Can you work these out from the model? Positions are in its coordinate system, mm. Face numbers are marked on the shaded views. A direction names the side the tool comes from. Coordinates: 2 decimals unless noted, no trailing zeros. Order: outer loops, then holes, each group sorted by start corner. A loop starts at its lowest first (then second) coordinate and runs counter-clockwise, first axis right, second up. Notation, with made-up numbers: M 48.5,61 L 59.5,61 A27 cw 59.5,77 Z; hole C 32,1 d5. An arc over 180 degrees is marked long. Answer as CSV lines item,"result". Start each with the question number.
1. If we section it at A-A (z = 4): List the corners of the cut face in (x, y) for me, plus the area to 3 significant figures.
2. On a 3-axis mill with a long thin cutter (end or side, diameter ignored), from which of +Z, -Z, +X, -X, +Y, -Y can I reach the whole of each face in a straight line? I mean the marked faces 1 and 2. Say none if no direction works.
3. If we section it at C-C (y = 23.5): List the corners of the cut face in (x, z) for me, plus the area to 3 significant figures.
4. If we section it at B-B (x = 30): List the corners of the cut face in (y, z) for me.
5. I need wall thicknesses on line 1 along Y through (x, z) = (38.5, 9.25); line 2 along X through (y, z) = (12.5, 11). Which ranges of each line are inside material? Lowest first, please. Write a range as from..to.
6. Will these pins go through, and if not, where does the flat tip stop? pin 1 (5 mm diameter, centred on x = 43, z = 10.5, fed in from -Y); pin 2 (6 mm diameter, centred on y = 5.5, z = 8, fed in from -X).
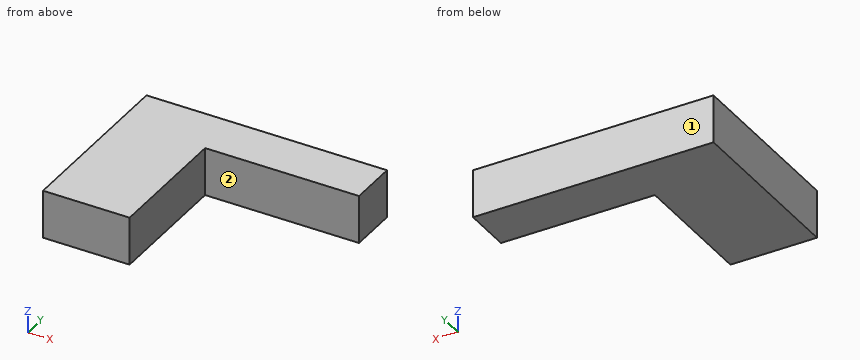
```python
from build123d import *

# Parameters (mm, degrees)
BOX001_W     = 32
BOX001_H     = 10
BOX001_DEPTH = 10
BOX_W        = 18
BOX_H        = 37
BOX_DEPTH    = 10


with BuildPart() as cubo001:
    # Box001 → Box001 (new body)
    with BuildSketch(Plane(origin=(18, 27, 0), x_dir=(1, 0, 0), z_dir=(0, 0, 1))):
        with Locations((16, 5)):
            Rectangle(BOX001_W, BOX001_H)
    extrude(amount=BOX001_DEPTH)


with BuildPart() as base:
    # Box → Box (new body)
    with BuildSketch(Plane.XY):
        with Locations((9, 18.5)):
            Rectangle(BOX_W, BOX_H)
    extrude(amount=BOX_DEPTH)

    # Fusion: union Cubo001
    add(cubo001.part)


with BuildPart() as base_1:
    # Fusion placement: moved
    add(base.part.moved(Location((0, 0, 2))))


solid = base_1.part
```
Solved:
1,outline,"M 0,0 L 18,0 L 18,27 L 50,27 L 50,37 L 0,37 Z"
1,area,"986 mm²"
2,face 1,"+Z, -Z, +X, -X, +Y"
2,face 2,"+Z, -Z, +X, -Y"
3,outline,"M 0,2 L 18,2 L 18,12 L 0,12 Z"
3,area,"180 mm²"
4,outline,"M 27,2 L 37,2 L 37,12 L 27,12 Z"
5,line 1,"27..37"
5,line 2,"0..18"
6,pin 1,"y = 27"
6,pin 2,"x = 0"
